```python
from build123d import *

# Parameters (mm, degrees)
SKETCH1_W                 = 41.8
SKETCH1_H                 = 143.8
BOSS_EXTRUDE1_DEPTH       = 12
SHELL1_T                  = -7
SHELL1_THICKNESS_2_FACE_W = 27.8
SHELL1_THICKNESS_2_FACE_H = 129.8
SHELL1_THICKNESS_2_DEPTH  = 4
SKETCH2_R                 = 2.2
CUT_EXTRUDE1_DEPTH        = 5.2
SKETCH3_R                 = 2.2
CUT_EXTRUDE2_DEPTH        = 5.2
SKETCH5_R                 = 1.7
CUT_EXTRUDE3_DEPTH        = 10
CHAMFER1_SIZE             = 2


with BuildPart() as part:
    # Sketch1 → Boss-Extrude1 (new body)
    with BuildSketch(Plane.XY):
        with Locations((0, 71.9)):
            Rectangle(SKETCH1_W, SKETCH1_H)
    extrude(amount=-BOSS_EXTRUDE1_DEPTH)

    # Shell1
    shell1_openings = [part.faces().sort_by_distance(p)[0] for p in [
        (0, 71.9, -12),
    ]]
    offset(amount=SHELL1_T, openings=shell1_openings, kind=Kind.INTERSECTION)

    # Shell1 thickness 2 face (on inner face of the shell) → Shell1 thickness 2 (cut)
    with BuildSketch(Plane(origin=(0, 71.9, -7), x_dir=(1, 0, 0), z_dir=(0, 0, 1))):
        Rectangle(SHELL1_THICKNESS_2_FACE_W, SHELL1_THICKNESS_2_FACE_H)
    extrude(amount=SHELL1_THICKNESS_2_DEPTH, mode=Mode.SUBTRACT)

    # Sketch2 → Cut-Extrude1 (cut)
    with BuildSketch(Plane(origin=(0, 143.8, 0), x_dir=(1, 0, 0), z_dir=(0, 1, 0))):
        with Locations(Location((-15, 6, 0), (0, 0, 270))):
            Circle(SKETCH2_R)
        with Locations(Location((15, 6, 0), (0, 0, 270))):
            Circle(SKETCH2_R)
    cut_extrude1 = extrude(amount=-CUT_EXTRUDE1_DEPTH, mode=Mode.SUBTRACT)

    # Mirror1: Cut-Extrude1 across plane
    add(cut_extrude1.mirror(Plane.ZX.offset(71.9)), mode=Mode.SUBTRACT)

    # Sketch3 → Cut-Extrude2 (cut)
    with BuildSketch(Plane.ZY.offset(20.9)):
        with Locations((-6, 129.4)):
            Circle(SKETCH3_R)
        with Locations((-6, 14.4)):
            Circle(SKETCH3_R)
    extrude(amount=-CUT_EXTRUDE2_DEPTH, mode=Mode.SUBTRACT)

    # Sketch5 → Cut-Extrude3 (cut)
    with BuildSketch(Plane(origin=(0, 0, -3), x_dir=(-1, 0, 0), z_dir=(0, 0, -1))):
        with Locations((-5.75, 63.9)):
            Circle(SKETCH5_R)
        with Locations((-5.75, 79.9)):
            Circle(SKETCH5_R)
    extrude(amount=-CUT_EXTRUDE3_DEPTH, mode=Mode.SUBTRACT)

    # Chamfer1
    chamfer1_edges = [part.edges().sort_by_distance(p)[0] for p in [
        (7.45, 63.9, 0),
        (7.45, 79.9, 0),
    ]]
    chamfer(chamfer1_edges, length=CHAMFER1_SIZE)


solid = part.part
```
Check sheet for the modelled part. Datum: model origin and axes. Units: mm. A direction names the side the tool comes from. Give positions to 0.01 mm unless a question says otherwise; leave off trailing zeros. Write each loop counter-clockwise with the first axis right and the second up, starting at its lowest first coordinate (ties: lowest second). Pieces come first, ordered by that corner, then holes. Notation, with made-up numbers: (61.25, 16) - (96.25, 16) arc R18 cw to (96.25, 44) - close; hole circle Ø9 at (24.5, 63.25). An arc over 180 degrees is marked (long way). Answer as a JSON object with one key per item and string values. Group by question number.
1) Sectioned sample at B-B (z = -10). Record the cut outline in (x, y), then the cut area to 3 significant figures.
2) Thickness scan on probe 1 along X at (y, z) = (140.85, -6); probe 2 along Y at (x, z) = (-19.35, -6); probe 3 along Y at (x, z) = (5.75, -2.4). Record the ranges inside material, lowest first. Write a range as from..to.
3) Depth check by flat-ended pin: P1, Ø1.3, axis at x = -14.5, z = -5.5, coming from the -Y side; P2, Ø2, axis at x = 5.75, y = 79.9, coming from the -Z side; P3, Ø3.5, axis at x = -15, z = -6, coming from the +Y side; P4, Ø4, axis at x = 5.75, y = 63.9, coming from the -Z side. Enter the tip coordinate at first touch or a pass-through.
4) Release check for a two-part mould opening along Z. For faces 4 (the face through (-14.2, 88.9, -12)), 5 (the face through (-15.843, 141.236, -3.968)), 6 (the face through (0, 136.8, -7)) record: pulls with the +Z half, pulls with the -Z half, needs draft (parallel to the pull), parting line crosses it, or undercut.
5) Sectioned sample at D-D (x = -8.5). Record the cut outline in (y, z).
6) Sectioned sample at C-C (y = 104.5). Record the cut outline in (x, z), then the cut area to 3 significant figures.
7) Sectioned sample at A-A (y = 79.9). Record the cut outline in (x, z), then the cut area to 3 significant figures.
8) Access from +Z, -Z, +X, -X, +Y, -Y to the whole of each face (thin tool, end or side, straight path). Record for faces 1 (the face through (-13.9, 71, -7)), 2 (the face through (15.66, 2.56, -3.9)), 3 (the face through (-15, 138.6, -6)).
Geometry results:
{
 "1": {"outline": "(-20.9, 0) - (20.9, 0) - (20.9, 143.8) - (-20.9, 143.8) - close; hole (-13.9, 7) - (13.9, 7) - (13.9, 136.8) - (-13.9, 136.8) - close", "area": "2,400 mm^2"},
 "2": {"probe 1": "x = -20.9..-17.2, -12.8..12.8, 17.2..20.9", "probe 2": "y = 0..12.2, 16.6..127.2, 131.6..143.8", "probe 3": "y = 0..62.2, 65.6..78.2, 81.6..143.8"},
 "3": {"P1": "stops at y = 5.2", "P2": "passes through", "P3": "stops at y = 138.6", "P4": "stops at z = -3"},
 "4": {"face 4": "pulls with the -Z half", "face 5": "undercut", "face 6": "needs draft"},
 "5": {"outline": "(0, -12) - (7, -12) - (7, -3) - (136.8, -3) - (136.8, -12) - (143.8, -12) - (143.8, 0) - (0, 0) - close"},
 "6": {"outline": "(-20.9, -12) - (-13.9, -12) - (-13.9, -3) - (13.9, -3) - (13.9, -12) - (20.9, -12) - (20.9, 0) - (-20.9, 0) - close", "area": "251 mm^2"},
 "7": {"outline": "(-20.9, -12) - (-13.9, -12) - (-13.9, -3) - (4.05, -3) - (4.05, -2) - (2.05, 0) - (-20.9, 0) - close; (7.45, -3) - (13.9, -3) - (13.9, -12) - (20.9, -12) - (20.9, 0) - (9.45, 0) - (7.45, -2) - close", "area": "237 mm^2"},
 "8": {"face 1": "-Z", "face 2": "-Y", "face 3": "+Y"}
}
